Here's how the part is built. I have some questions about the finished solid (model axes, mm). Face numbers are marked on the shaded views. A direction names the side the tool comes from. Coordinates: 2 decimals unless noted, no trailing zeros. Write each loop counter-clockwise with the first axis right and the second up, starting at its lowest first coordinate (ties: lowest second). Pieces come first, ordered by that corner, then holes.
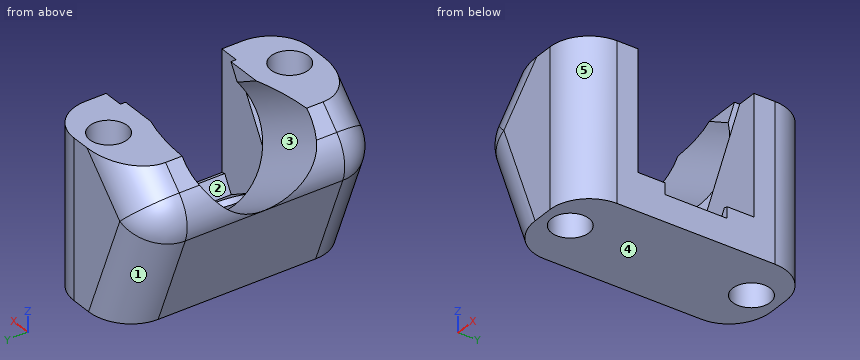
```python
from build123d import *

# Parameters (mm, degrees)
F1_DEPTH       = 15
F1_DEPTH_BACK  = 15
F6_R           = 5
F5_R           = 2.38125
F7_DEPTH       = 25
F7_DEPTH_BACK  = 25
F10_DEPTH      = 9.3
F11_START      = -9.3
F11_DEPTH      = 15.7
F12_SIZE       = 1
F14_R          = 3
F16_DEPTH      = 2.5
F15_W          = 5.334
F15_H          = 7.923
F17_DEPTH      = 25
F17_DEPTH_BACK = 2.5


with BuildPart() as f1:
    # F0 (on Front) → F1 (new body, two sides)
    with BuildSketch(Plane.XZ) as f1_sk:
        Polygon((-13, -10.8026722446), (0, -10.8026722446), (0, 9.1973277554), (-14.3321100622, 9.1973277554), (-19.0368395666, 4.3939077003), align=None)
    extrude(amount=F1_DEPTH)
    extrude(f1_sk.sketch, amount=-F1_DEPTH_BACK)

    # F6
    f6_edges = [f1.edges().sort_by_distance(p)[0] for p in [
        (-19.03684, 0, 4.393908),
        (-16.01842, -15, -3.204382),
        (-16.01842, 15, -3.204382),
        (-16.684475, -15, 6.795618),
        (-16.684475, 15, 6.795618),
        (0, -15, -0.802672),
        (0, 15, -0.802672),
    ]]
    fillet(f6_edges, radius=F6_R)

    # F5 (on Top) → F7 (cut, two sides)
    with BuildSketch(Plane.XY) as f7_sk:
        with Locations((-6.2674125656, -11.5)):
            Circle(F5_R)
        with Locations((-6.2674125656, 11.5)):
            Circle(F5_R)
    extrude(amount=-F7_DEPTH, mode=Mode.SUBTRACT)
    extrude(f7_sk.sketch, amount=F7_DEPTH_BACK, mode=Mode.SUBTRACT)

    # F9 (on face) → F10 (cut)
    with BuildSketch(Plane(origin=(2.1650635095, 0, -1.25), x_dir=(0, 1, 0), z_dir=(0.8660254038, 0, -0.5))):
        Polygon((-7.35, -7.6351069248), (7.35, -7.6351069248), (7.35, 8.0451745412), (7.35, 12.5973122194), (-7.35, 12.5973122194), (-7.35, 8.0451745412), align=None)
    extrude(amount=-F10_DEPTH, mode=Mode.SUBTRACT)

    # F8 (on face) → F11 (cut)
    with BuildSketch(Plane(origin=(2.1650635095, 0, -1.25), x_dir=(0, 1, 0), z_dir=(0.8660254038, 0, -0.5)).offset(F11_START)):
        with BuildLine():
            Line((-6.6921999912, 12.0207928121), (-6.6921999912, 4.4500407902))
            ThreePointArc((-6.6921999912, 4.4500407902), (0, -7.7199661918), (6.6921999912, 4.4500407902))
            Line((6.6921999912, 4.4500407902), (6.6921999912, 12.0207928121))
            Line((6.6921999912, 12.0207928121), (-6.6921999912, 12.0207928121))
        make_face()
    extrude(amount=-F11_DEPTH, mode=Mode.SUBTRACT)

    # F12
    f12_edges = [f1.edges().sort_by_distance(p)[0] for p in [
        (0, 0, -5),
    ]]
    chamfer(f12_edges, length=F12_SIZE)

    # F14 (on face) → F16 (cut)
    with BuildSketch(Plane(origin=(-3.8175534624, 0, -6.6121965575), x_dir=(0.8660254038, 0, -0.5), z_dir=(-0.5, 0, -0.8660254038))):
        with Locations((-1.596442773, 4.0683373809)):
            Circle(F14_R)
    extrude(amount=F16_DEPTH, mode=Mode.SUBTRACT)

    # F15 (on face) → F17 (cut, two sides)
    with BuildSketch(Plane(origin=(-3.8175534624, 0, -6.6121965575), x_dir=(0.8660254038, 0, -0.5), z_dir=(-0.5, 0, -0.8660254038))) as f17_sk:
        with Locations((1.0496865725, 0)):
            Rectangle(F15_W, F15_H)
    extrude(amount=-F17_DEPTH, mode=Mode.SUBTRACT)
    extrude(f17_sk.sketch, amount=F17_DEPTH_BACK, mode=Mode.SUBTRACT)


solid = f1.part
```
1) On a 3-axis mill with a long thin cutter (end or side, diameter ignored), from which of +Z, -Z, +X, -X, +Y, -Y can I reach the whole of each face in a straight line? I mean the marked faces 1 and 2. Say none if no direction works.
Values follow:
face 1: -Z, -X, +Y
face 2: +Z
2) Imagine slicing it at B-B on x = -1.25. Please give me the cut outline in (y, z), then the cut area to 3 significant figures.
Values follow:
outline: (-13.31, -10.8) - (13.31, -10.8) - (13.31, 9.2) - (7.35, 9.2) - (7.35, -7.17) - (3.96, -7.17) - (3.96, -9.6) - (-3.96, -9.6) - (-3.96, -7.17) - (-7.35, -7.17) - (-7.35, 9.2) - (-13.31, 9.2) - close
area: 272 mm2
3) Imagine slicing it at D-D on z = -0.5. Count the separate pieces of the cut face and the enclosed holes in it, then the cut area to 3 significant figures.
Values follow:
separate pieces: 1
enclosed holes: 2
area: 278 mm2
4) Imagine slicing it at C-C on y = 12.5. Please give me the cut outline in (x, z).
Values follow:
outline: (-17.21, 1.62) - (-12.28, -10.8) - (-8.43, -10.8) - (-8.43, 9.2) - (-13.39, 9.2) - (-16.28, 6.25) arc R4.33 ccw to start; (-4.11, -10.8) - (-0.67, -10.8) - (-0.67, 9.2) - (-4.11, 9.2) - close
5) Will these pins go through, and if not, where does the flat tip stop? pin 1 (1 mm diameter, centred on x = -2, z = 7, fed in from +Y); pin 2 (4 mm diameter, centred on x = -11, z = 6.5, fed in from -Y); pin 3 (3 mm diameter, centred on x = -6.27, y = -11.5, fed in from -Z); pin 4 (3 mm diameter, centred on x = -11.5, z = -7.5, fed in from +Y).
Values follow:
pin 1: stops at y = 14.33
pin 2: stops at y = -15
pin 3: passes through
pin 4: stops at y = 14.92
6) Imagine slicing it at A-A on y = -11.5. Please give me the cut outline in (x, z).
Values follow:
outline: (-17.62, 1.46) - (-12.75, -10.8) - (-8.65, -10.8) - (-8.65, 9.2) - (-14.01, 9.2) - (-16.6, 6.56) arc R4.77 ccw to start; (-3.89, -10.8) - (-0.23, -10.8) - (-0.23, 9.2) - (-3.89, 9.2) - close
7) I need wall thicknesses on probe 1 along Y at (x, z) = (-6.25, 1.5); probe 2 along Y at (x, z) = (-8.25, 7.5); probe 3 along X at (y, z) = (-11.5, 5). Which ranges of each line are inside material? Lowest first, please.
Values follow:
probe 1: y = -15 to -13.88, -9.12 to -7.35, 7.35 to 9.12, 13.88 to 15
probe 2: y = -15 to -12.82, -10.18 to -7.62, 7.62 to 10.18, 12.82 to 15
probe 3: x = -17.61 to -8.65, -3.89 to -0.23
8) We'd pull the mould along X, two halves only. Please class the marked faces 3, 4 and 5: pulls with the +X half, pulls with the -X half, needs draft (parallel to the pull), parting line crosses it, or undercut.
Values follow:
face 3: undercut
face 4: needs draft
face 5: pulls with the +X half
